Geometry: final body of the model. Coordinates: model frame, mm. A direction names the side the tool comes from. Round coordinates to 2 decimals unless told otherwise and drop trailing zeros. Loops run counter-clockwise (first coordinate to the right, second up) from the corner with the lowest first, then second, coordinate; pieces in that order, holes last. Notation, with made-up numbers: (24, 61) -> (79, 61) arc R33 ccw to (79, 99) -> close; hole circle Ø11 at (83.25, 60.25). An arc over 180 degrees is marked (long way). Answer in a Markdown table with one row per item.
```python
from build123d import *

# Parameters (mm, degrees)
SKETCH1_R           = 14.2875
BOSS_EXTRUDE1_DEPTH = 12.7
FILLET1_R           = 2.032
SHELL1_T            = -2.54
CUT_EXTRUDE1_REACH  = 25.865
SKETCH2_R           = 0.0127


with BuildPart() as part:
    # Sketch1 → Boss-Extrude1 (new body)
    with BuildSketch(Plane(origin=(0, 0, 0), x_dir=(1, 0, 0), z_dir=(0, 1, 0))):
        with Locations(Location((0, 0, 0), (0, 0, 270))):
            Circle(SKETCH1_R)
    extrude(amount=BOSS_EXTRUDE1_DEPTH)

    # Fillet1
    fillet1_edges = [part.edges().sort_by_distance(p)[0] for p in [
        (0, 12.7, -14.2875),
    ]]
    fillet(fillet1_edges, radius=FILLET1_R)

    # Shell1
    shell1_openings = [part.faces().sort_by_distance(p)[0] for p in [
        (0, 0, 0),
    ]]
    offset(amount=SHELL1_T, openings=shell1_openings, kind=Kind.INTERSECTION)

    # Sketch2 → Cut-Extrude1 (cut, up to next)
    with BuildSketch(Plane(origin=(0, 12.7, 0), x_dir=(1, 0, 0), z_dir=(0, 1, 0)), mode=Mode.PRIVATE) as cut_extrude1_sk1:
        with Locations(Location((0, 0, 0), (0, 0, 270))):
            Circle(SKETCH2_R)
    cut_extrude1_tool1 = extrude(cut_extrude1_sk1.sketch, amount=-CUT_EXTRUDE1_REACH, mode=Mode.PRIVATE) & part.part
    add(cut_extrude1_tool1.solids().sort_by_distance((0, 12.7, 0))[0], mode=Mode.SUBTRACT)


solid = part.part
```
Item 1: Set-up query: faces 1 (the flat face through (0.2, 10.16, -0.2)), 2 (the flat face through (-12, 0, -2)). Return all of +Z, -Z, +X, -X, +Y, -Y with unobstructed straight access to the full face (end or side cutting, diameter ignored); none if empty.
Ans:
| item | result |
|---|---|
| face 1 | -Y |
| face 2 | +Z, -Z, +X, -X, -Y |
Item 2: First-contact query: P1, Ø1, axis at y = 5, z = 10.5, coming from the -X side; P2, Ø2, axis at x = 7.5, y = 3, coming from the -Z side; P3, Ø6, axis at x = -10, y = 10, coming from the +Z side. Flat tips, straight axial feed; report the tip coordinate or a pass-through.
Ans:
| item | result |
|---|---|
| P1 | x = -10.2 |
| P2 | z = -12.72 |
| P3 | z = 12.46 |
Item 3: Section query A-A, the plane y = 2.5. Output: boundary loops of the cut face in (x, z) (1 decimal).
Ans:
| item | result |
|---|---|
| outline | circle Ø28.6 at (0, 0); hole circle Ø23.5 at (0, 0) |
Item 4: Ray query, L1, parallel to X at y = 3, z = 0; L2, parallel to Y at x = 7.5, z = -9; L3, parallel to X at y = 1.75, z = -10. Return the intervals inside material, ascending.
Ans:
| item | result |
|---|---|
| L1 | -14.29 to -11.75, 11.75 to 14.29 |
| L2 | 10.16 to 12.7 |
| L3 | -10.2 to -6.16, 6.16 to 10.2 |
Item 5: Section query B-B, the plane y = 11.5. Output: boundary loops of the cut face in (x, z).
Ans:
| item | result |
|---|---|
| outline | circle Ø28.22 at (0, 0); hole circle Ø0.03 at (0, 0) |
